Drawing for the job (mm, zero at the part's lowest x, y, z). A direction names the side the tool comes from. Round coordinates to 2 decimals unless told otherwise and drop trailing zeros. Loops run counter-clockwise (first coordinate to the right, second up) from the corner with the lowest first, then second, coordinate; pieces in that order, holes last. Notation, with made-up numbers: (68.25, -23.75) -> (84.25, -23.75) arc R16 ccw to (84.25, -14.75) -> close; hole circle Ø11 at (-12, 68). An arc over 180 degrees is marked (long way). Put each result on its own line as item: value. Start each with the question number.
Item 1: Cut at C-C, the plane z = 43.5. List the corners of the cut face in (x, y) (1 decimal), plus the area to 3 significant figures.
Item 2: Cut at A-A, the plane x = 4.5. List the corners of the cut face in (y, z).
Item 3: Drill centre lines: probe 1 along Z at (x, y) = (5, 40.5); probe 2 along X at (y, z) = (23, 40); probe 3 along X at (y, z) = (17, 32) (1 decimal). Where is each one in solid material? Low to high. Write a range as [from, to].
Item 4: Cut at B-B, the plane y = 33. List the corners of the cut face in (x, z), plus the area to 4 significant figures.
Item 5: Flat gauge pins, fed straight in: pin 1 Ø1 at (x, z) = (15.5, 61) entering from +Y; pin 2 Ø1.5 at (y, z) = (15, 12) entering from +X; pin 3 Ø2 at (x, z) = (13.5, 69.5) entering from +Y. Where does each tip first touch, or does it go through?
Item 6: Cut at D-D, the plane x = 35.5. List the corners of the cut face in (y, z), plus the area to 3 significant figures.
Item 7: Tool access for the marked faces 1 and 2: list every direction of +Z, -Z, +X, -X, +Y, -Y with a clear straight run to the whole face (end or side of a thin tool).
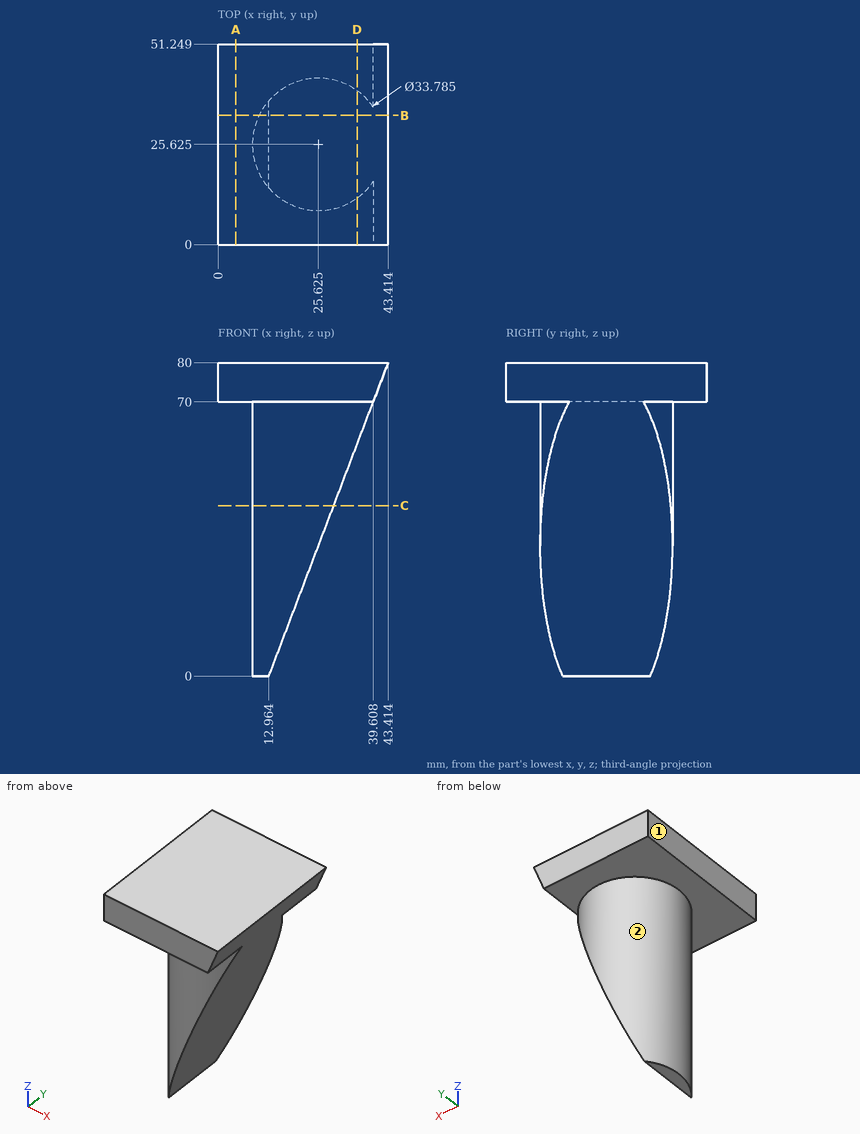
Reply:
1. outline: (29.5, 9.2) -> (29.5, 42.1) arc R16.9 ccw (long way) to start
1. area: 579 mm^2
2. outline: (0, 70) -> (51.25, 70) -> (51.25, 80) -> (0, 80) -> close
3. probe 1: z = [70, 80]
3. probe 2: x = [8.94, 28.19]
3. probe 3: x = [11.1, 25.1]
4. outline: (0, 70) -> (10.43, 70) -> (10.43, 0) -> (12.96, 0) -> (43.41, 80) -> (0, 80) -> close
4. area: 1,525 mm^2
5. pin 1: stops at y = 39.51
5. pin 2: stops at x = 17.82
5. pin 3: stops at y = 51.25
6. outline: (0, 70) -> (11.92, 70) -> (11.92, 59.21) -> (39.33, 59.21) -> (39.33, 70) -> (51.25, 70) -> (51.25, 80) -> (0, 80) -> close
6. area: 808 mm^2
7. face 1: +Z, -Z, -X, +Y, -Y
7. face 2: -Z
